from build123d import *

# Parameters (mm, degrees)
SKETCH_1_R          = 6.15
EXTRUDE_1_DEPTH     = 15
EXTRUDE_2_DEPTH     = 30
SKETCH_3_R          = 7
EXTRUDE_3_DEPTH     = 3
SKETCH_4_R          = 5
CUT_EXTRUDE_1_DEPTH = 10
M5X0_8_1_REACH      = 53.556
M5X0_8_1_BORE_R     = 2.1


with BuildPart() as part:
    # 草图1 → 凸台-拉伸1 (new body)
    with BuildSketch(Plane.XY):
        Circle(SKETCH_1_R)
    extrude(amount=EXTRUDE_1_DEPTH)

    # 草图2 → 凸台-拉伸2 (add)
    with BuildSketch(Plane.XY.offset(15)):
        Polygon((6.373936419, 5.862843552), (-1.890403245, 8.451412638), (-8.264339665, 2.588569085), (-6.373936419, -5.862843552), (1.890403245, -8.451412638), (8.264339665, -2.588569085), align=None)
    extrude(amount=EXTRUDE_2_DEPTH)

    # 草图3 → 凸台-拉伸3 (add)
    with BuildSketch(Plane.XY.offset(45)):
        Circle(SKETCH_3_R)
    extrude(amount=EXTRUDE_3_DEPTH)

    # 草图4 → 切除-拉伸1 (cut)
    with BuildSketch(Plane.XY.offset(48)):
        Circle(SKETCH_4_R)
    extrude(amount=-CUT_EXTRUDE_1_DEPTH, mode=Mode.SUBTRACT)

    # M5x0.8 螺纹孔1 bore → M5x0.8 螺纹孔1 (cut, up to next)
    with BuildSketch(Plane(origin=(2.241766587, 7.157128095, 0), x_dir=(-0.9542837460036324, 0.2989022116232579, 0), z_dir=(0.2989022116232579, 0.9542837460036325, 0)), mode=Mode.PRIVATE) as m5x0_8_1_sk1:
        with Locations((0, 40.158364076)):
            Circle(M5X0_8_1_BORE_R)
    m5x0_8_1_tool1 = extrude(m5x0_8_1_sk1.sketch, amount=-M5X0_8_1_REACH, mode=Mode.PRIVATE) & part.part
    add(m5x0_8_1_tool1.solids().sort_by_distance((2.241767, 7.157128, 40.158364))[0], mode=Mode.SUBTRACT)


solid = part.part
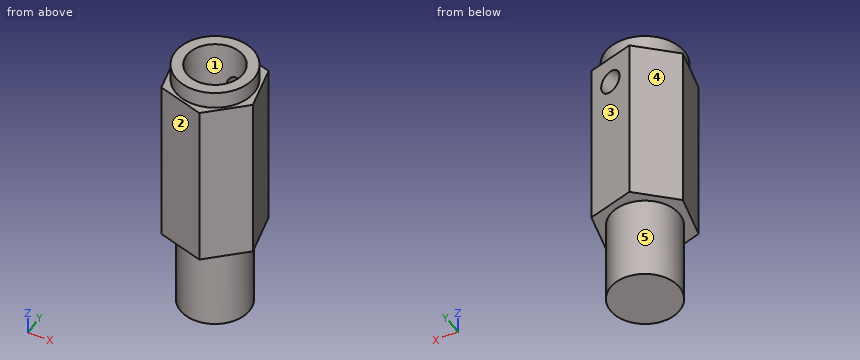
Can you work these out from the model? Positions are in its coordinate system, mm. Face numbers are marked on the shaded views. A direction names the side the tool comes from. Coordinates: 2 decimals unless noted, no trailing zeros. Order: outer loops, then holes, each group sorted by start corner. A loop starts at its lowest first (then second) coordinate and runs counter-clockwise, first axis right, second up. Notation, with made-up numbers: M 9,-26 L 33,-26 A28 cw 33,-3 Z; hole C 24.5,-29.5 d4. An arc over 180 degrees is marked long. Answer as CSV lines item,"result".
(1) Please list where these lines run through material, in increasing order: L1, parallel to Y at x = 0, z = 46; L2, parallel to Z at x = -7.25, y = 0; L3, parallel to Z at x = -0.75, y = -6.25.
Geometry check:
L1,"-7 to -5, 5 to 7"
L2,"15 to 45"
L3,"15 to 48"
(2) Suppose I cut it at C-C on x = -3.25. Please give me the cut outline in (y, z).
Geometry check:
outline,"M -6.84,15 L -5.22,15 L -5.22,0 L 5.22,0 L 5.22,15 L 7.2,15 L 7.2,45 L 6.2,45 L 6.2,48 L 3.8,48 L 3.8,38 L -3.8,38 L -3.8,48 L -6.2,48 L -6.2,45 L -6.84,45 Z"
(3) Suppose I cut it at A-A on y = -3.5. Please give me the cut outline in (x, z), plus the area to 3 significant figures.
Geometry check:
outline,"M -6.9,15 L -5.06,15 L -5.06,0 L 5.06,0 L 5.06,15 L 7.27,15 L 7.27,45 L 6.06,45 L 6.06,48 L 3.57,48 L 3.57,38 L -3.57,38 L -3.57,48 L -6.06,48 L -6.06,45 L -6.9,45 Z"
area,"542 mm^2"
(4) On a 3-axis mill with a long thin cutter (end or side, diameter ignored), from which of +Z, -Z, +X, -X, +Y, -Y can I reach the whole of each face in a straight line? I mean the marked faces 4 and 5. Say none if no direction works.
Geometry check:
face 4,"+Z, -Z, -X, +Y"
face 5,"-Z"
(5) Suppose I cut it at B-B on z = 27.5. Please give me the cut outline in (x, y), plus the area to 3 significant figures.
Geometry check:
outline,"M -8.26,2.59 L -6.37,-5.86 L 1.89,-8.45 L 8.26,-2.59 L 6.37,5.86 L -1.89,8.45 Z"
area,"195 mm^2"
(6) I'm going to push flat-ended pins straight in: pin 1 (1.5 mm diameter, centred on x = -4, z = 16.5, fed in from -Y); pin 2 (4 mm diameter, centred on y = 2.5, z = 14.5, fed in from +X); pin 3 (8 mm diameter, centred on y = -3, z = 25, fed in from -X). Where does each tip first touch, or does it pass through?
Geometry check:
pin 1,"y = -6.84"
pin 2,"x = 7.56"
pin 3,"x = -7.91"
(7) If we mould it in two halves opening along X, with no side actions, what happens to the marked faces 1, 2 and 3? For each: released by +X, released by -X, zero draft, split by the parting line, or undercut.
Geometry check:
face 1,"undercut"
face 2,"released by -X"
face 3,"released by +X"
(8) Suppose I cut it at D-D on z = 9. Please give me the cut outline in (x, y).
Geometry check:
outline,"C 0,0 d12.3"
